```python
from build123d import *

# Parameters (mm, degrees)
SKETCH1_R           = 2
BOSS_EXTRUDE1_DEPTH = 33
SKETCH1_3_W         = 53
SKETCH1_3_H         = 12
BOSS_EXTRUDE2_DEPTH = 21
BOSS_EXTRUDE3_DEPTH = 8


with BuildPart() as part:
    # Sketch1 → Boss-Extrude1 (new body)
    with BuildSketch(Plane(origin=(0, 0, 0), x_dir=(1, 0, 0), z_dir=(0, 1, 0))):
        Polygon((43.5, -30), (43.5, 30), (16.5, 30), (16.5, 18), (-36.5, 18), (-36.5, 30), (-62.5, 30), (-62.5, -30), (-36.5, -30), (-36.5, -18), (16.5, -18), (16.5, -30), align=None)
        with Locations(Location((-55, -24, 0), (0, 0, 270))):
            Circle(SKETCH1_R, mode=Mode.SUBTRACT)
        with Locations(Location((34, -24, 0), (0, 0, 270))):
            Circle(SKETCH1_R, mode=Mode.SUBTRACT)
        with Locations(Location((-55, 24, 0), (0, 0, 270))):
            Circle(SKETCH1_R, mode=Mode.SUBTRACT)
        with Locations(Location((34, 24, 0), (0, 0, 270))):
            Circle(SKETCH1_R, mode=Mode.SUBTRACT)
    extrude(amount=BOSS_EXTRUDE1_DEPTH)

    # Sketch1_3 → Boss-Extrude2 (add)
    with BuildSketch(Plane(origin=(0, 0, 0), x_dir=(1, 0, 0), z_dir=(0, 1, 0))):
        with Locations((-10, -24)):
            Rectangle(SKETCH1_3_W, SKETCH1_3_H)
        with Locations((-10, 24)):
            Rectangle(SKETCH1_3_W, SKETCH1_3_H)
    extrude(amount=BOSS_EXTRUDE2_DEPTH)

    # Sketch1_4 → Boss-Extrude3 (add)
    with BuildSketch(Plane(origin=(0, 0, 0), x_dir=(1, 0, 0), z_dir=(0, 1, 0))):
        with BuildLine():
            Line((54.5, 30), (43.5, 30))
            Line((43.5, 30), (43.5, -30))
            Line((43.5, -30), (54.5, -30))
            Line((54.5, -30), (54.5, -26))
            ThreePointArc((54.5, -26), (52.5, -24), (54.5, -22))
            Line((54.5, -22), (54.5, 22))
            ThreePointArc((54.5, 22), (52.5, 24), (54.5, 26))
            Line((54.5, 26), (54.5, 30))
        make_face()
        with BuildLine():
            Line((62.5, 30), (54.5, 30))
            Line((54.5, 30), (54.5, 26))
            ThreePointArc((54.5, 26), (55.914213562, 25.414213562), (56.5, 24))
            ThreePointArc((56.5, 24), (55.914213562, 22.585786438), (54.5, 22))
            Line((54.5, 22), (54.5, -22))
            ThreePointArc((54.5, -22), (55.914213562, -22.585786438), (56.5, -24))
            ThreePointArc((56.5, -24), (55.914213562, -25.414213562), (54.5, -26))
            Line((54.5, -26), (54.5, -30))
            Line((54.5, -30), (62.5, -30))
            Line((62.5, -30), (62.5, 30))
        make_face()
    extrude(amount=BOSS_EXTRUDE3_DEPTH)


solid = part.part
```
The model under review builds one solid part; all positions refer to its coordinate system, in mm. A direction names the side the tool comes from. Give positions to 0.01 mm unless a question says otherwise; leave off trailing zeros. Write each loop counter-clockwise with the first axis right and the second up, starting at its lowest first coordinate (ties: lowest second). Pieces come first, ordered by that corner, then holes. Notation, with made-up numbers: (8, -6) - (34, -6) arc R31 ccw to (34, 27) - close; hole circle Ø5 at (57.25, 24.25). An arc over 180 degrees is marked (long way). Answer in a Markdown table with one row per item. Add a question column.
1. Tool access review of faces 1 (the flat face through (-10, 21, -24)), 2 (the flat face through (-36.5, 27, 24)), 3 (the cylindrical face through (-53, 16, -24)), 4 (the flat face through (53, 8, 0)): name each direction out of +Z, -Z, +X, -X, +Y, -Y from which nothing blocks a thin tool from reaching the whole face with its end or side.
2. Insertion check: P1, Ø7.5, axis at y = 19.5, z = 3, coming from the +X side; P2, Ø4, axis at x = -24.5, z = 21, coming from the +Y side; P3, Ø9.5, axis at x = 2.5, y = 28.5, coming from the -Z side. Each pin has a flat end and moves straight along its axis. Give the tip position at first contact, or say it passes through.
3. We need section B-B on x = -3.5. Write out the cut boundary in (y, z), then the cut area to 3 significant figures.
4. We need section D-D on z = -13.5. Write out the cut boundary in (x, y).
5. We need section A-A on y = 23.5. Write out the cut boundary in (x, z).
6. Wall thickness on line 1 along X through (y, z) = (26, 24); line 2 along X through (y, z) = (17.5, 24); line 3 along X through (y, z) = (26, 25.5): over which ranges is each line inside the solid? List them lowest first. Write a range as [from, to].
7. Draft analysis for pull direction Z (two halves, no side actions). For faces 5 (the cylindrical face through (32, 16, -24)), 6 (the flat face through (1, 13, -30)), 7 (the flat face through (-10, 27, 18)), state which applies: +Z half, -Z half, draft (parallel to the pull), parting line (faces both ways), or undercut.
8. We need section C-C on x = -55. Write out the cut boundary in (y, z), then the cut area to 3 significant figures.
Ans:
| question | item | result |
|---|---|---|
| 1 | face 1 | -Z, +Y |
| 1 | face 2 | +Z, +Y |
| 1 | face 3 | +Y, -Y |
| 1 | face 4 | +Z, -Z, +X, +Y |
| 2 | P1 | stops at x = 43.5 |
| 2 | P2 | stops at y = 21 |
| 2 | P3 | stops at z = -18 |
| 3 | outline | (0, -30) - (21, -30) - (21, -18) - (33, -18) - (33, 18) - (21, 18) - (21, 30) - (0, 30) - close |
| 3 | area | 1,690 mm^2 |
| 4 | outline | (-62.5, 0) - (62.5, 0) - (62.5, 8) - (43.5, 8) - (43.5, 33) - (-62.5, 33) - close |
| 5 | outline | (-62.5, -30) - (-36.5, -30) - (-36.5, -18) - (16.5, -18) - (16.5, -30) - (43.5, -30) - (43.5, 30) - (16.5, 30) - (16.5, 18) - (-36.5, 18) - (-36.5, 30) - (-62.5, 30) - close; hole circle Ø4 at (-55, -24); hole circle Ø4 at (-55, 24); hole circle Ø4 at (34, -24); hole circle Ø4 at (34, 24) |
| 6 | line 1 | x = [-62.5, -57], [-53, -36.5], [16.5, 32], [36, 43.5] |
| 6 | line 2 | x = [-62.5, -57], [-53, 32], [36, 43.5] |
| 6 | line 3 | x = [-62.5, -56.32], [-53.68, -36.5], [16.5, 32.68], [35.32, 43.5] |
| 7 | face 5 | undercut |
| 7 | face 6 | -Z half |
| 7 | face 7 | +Z half |
| 8 | outline | (0, -30) - (33, -30) - (33, -26) - (0, -26) - close; (0, -22) - (33, -22) - (33, 22) - (0, 22) - close; (0, 26) - (33, 26) - (33, 30) - (0, 30) - close |
| 8 | area | 1,720 mm^2 |
